The model under review builds one solid part; all positions refer to its coordinate system, in mm. Face numbers are marked on the shaded views. A direction names the side the tool comes from. Round coordinates to 2 decimals unless told otherwise and drop trailing zeros. Write each loop counter-clockwise with the first axis right and the second up, starting at its lowest first coordinate (ties: lowest second). Pieces come first, ordered by that corner, then holes. Notation, with made-up numbers: M -37,68 L -1,68 A11 ccw -1,85 Z; hole C 0.25,38.5 d8. An arc over 180 degrees is marked long. Write item = value, one per line. Start each with the question number.
Item 1: Take a section at D-D, the plane x = 2. Give the boundary of the cut face in (y, z).
Item 2: The part is to be moulded in two halves that separate along Y. For the marked faces 1, 2, 3 and 4, say which applies: +Y half, -Y half, draft (parallel to the pull), parting line (faces both ways), or undercut.
Item 3: Take a section at A-A, the plane x = 16. Give the boundary of the cut face in (y, z).
Item 4: Take a section at B-B, the plane y = 4. Give the boundary of the cut face in (x, z), plus the area to 4 significant figures.
Item 5: Take a section at C-C, the plane z = -16. Give the boundary of the cut face in (x, y).
Item 6: Tool access review of the marked faces 5 and 6: name each direction out of +Z, -Z, +X, -X, +Y, -Y from which nothing blocks a thin tool from reaching the whole face with its end or side.
Item 7: To check wall thickness, follow line 1 along Y through (x, z) = (16, -13.5); line 2 along X through (y, z) = (6.5, -16.25); line 3 along Y through (x, z) = (-2, -12.75). State the ranges of each line that lie inside material, in increasing order.
Item 8: For pin 1 Ø2.5 at (x, y) = (-3.5, 4) entering from +Z, flat-tipped, find the tip position at first contact; note if it passes through.
from build123d import *

# Parameters (mm, degrees)
SKETCH1_W           = 21
SKETCH1_H           = 5.5
BOSS_EXTRUDE1_DEPTH = 8
SKETCH2_W           = 21
SKETCH2_H           = 5.1
CUT_EXTRUDE1_DEPTH  = 5.5
SKETCH3_R           = 1.5
CUT_EXTRUDE2_DEPTH  = 10


with BuildPart() as part:
    # Sketch1 → Boss-Extrude1 (new body)
    with BuildSketch(Plane(origin=(0, 0, 0), x_dir=(1, 0, 0), z_dir=(0, 1, 0))):
        Polygon((-20, 20), (-20, 12), (-10.5, 12), (-10.5, 17.5), (10.5, 17.5), (10.5, 12), (20, 12), (20, 20), align=None)
        with Locations((0, 14.75)):
            Rectangle(SKETCH1_W, SKETCH1_H)
    extrude(amount=BOSS_EXTRUDE1_DEPTH)

    # Sketch2 → Cut-Extrude1 (cut)
    with BuildSketch(Plane.XY.offset(-12)):
        with Locations((0, 4)):
            Rectangle(SKETCH2_W, SKETCH2_H)
    extrude(amount=-CUT_EXTRUDE1_DEPTH, mode=Mode.SUBTRACT)

    # Sketch3 → Cut-Extrude2 (cut)
    with BuildSketch(Plane(origin=(0, 0, -20), x_dir=(-1, 0, 0), z_dir=(0, 0, -1))):
        with Locations((-16, 4)):
            Circle(SKETCH3_R)
        with Locations((16, 4)):
            Circle(SKETCH3_R)
    extrude(amount=-CUT_EXTRUDE2_DEPTH, mode=Mode.SUBTRACT)


solid = part.part
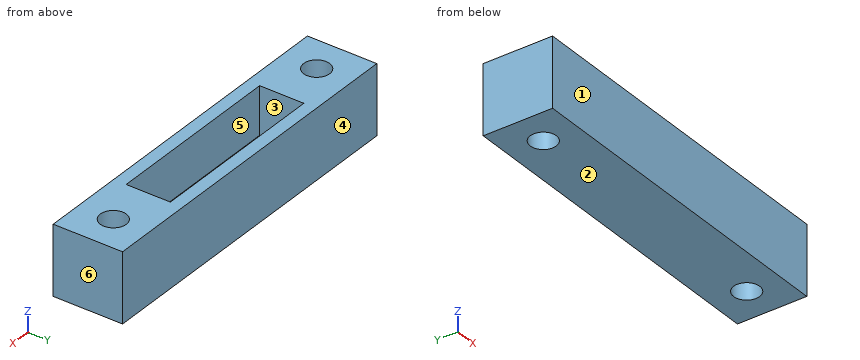
Response values:
q1.outline = M 0,-20 L 8,-20 L 8,-12 L 6.55,-12 L 6.55,-17.5 L 1.45,-17.5 L 1.45,-12 L 0,-12 Z
q2.face_1 = -Y half
q2.face_2 = draft
q2.face_3 = undercut
q2.face_4 = +Y half
q3.outline = M 0,-20 L 2.5,-20 L 2.5,-12 L 0,-12 Z; M 5.5,-20 L 8,-20 L 8,-12 L 5.5,-12 Z
q4.outline = M -20,-20 L -17.5,-20 L -17.5,-12 L -20,-12 Z; M -14.5,-20 L 14.5,-20 L 14.5,-12 L 10.5,-12 L 10.5,-17.5 L -10.5,-17.5 L -10.5,-12 L -14.5,-12 Z; M 17.5,-20 L 20,-20 L 20,-12 L 17.5,-12 Z
q4.area = 156.5 mm2
q5.outline = M -20,0 L 20,0 L 20,8 L -20,8 Z; hole C -16,4 d3; hole M -10.5,1.45 L 10.5,1.45 L 10.5,6.55 L -10.5,6.55 Z; hole C 16,4 d3
q6.face_5 = +Z
q6.face_6 = +Z, -Z, +X, +Y, -Y
q7.line_1 = 0 to 2.5, 5.5 to 8
q7.line_2 = -20 to -10.5, 10.5 to 20
q7.line_3 = 0 to 1.45, 6.55 to 8
q8.pin_1 = -17.5
